Part model, mm, in its own coordinate system. A direction names the side the tool comes from. Give positions to 0.01 mm unless a question says otherwise; leave off trailing zeros. Order: outer loops, then holes, each group sorted by start corner. A loop starts at its lowest first (then second) coordinate and runs counter-clockwise, first axis right, second up. Notation, with made-up numbers: (-17, 54.25) -> (-8, 54.25) arc R15 ccw to (-8, 71.25) -> close; hole circle Ø11 at (-21.75, 80). An arc over 180 degrees is marked (long way). Write item = value, one per line. Start each with the question number.
Item 1: Band-saw the part on C-C on y = 6.25. Write the cut outline in (x, z).
Item 2: Band-saw the part on A-A on y = 3.75. Write the cut outline in (x, z).
Item 3: Pull direction Z, two halves, no side cores. Call faces 1 (the face through (-1, 7, 3)), 2 (the face through (-1, 6, 2)), 3 (the face through (-2, 6.3, 2.4)), 4 (the face through (-15, 6.7, 0.4)): +Z half, -Z half, draft (parallel to the pull), parting line (faces both ways), or undercut.
Item 4: Band-saw the part on B-B on z = 1.7. Write the cut outline in (x, y), plus the area to 3 significant figures.
Item 5: Flat gauge pins, fed straight in: P1, Ø0.9, axis at x = -9, z = 2, coming from the -Y side; P2, Ø1.2, axis at y = 7, z = 2, coming from the -X side. Where does each tip first touch, or does it go through?
Item 6: Band-saw the part on D-D on z = 0.3. Write the cut outline in (x, y), plus the area to 3 significant figures.
Item 7: Tool access for faces 5 (the face through (-9, 4, 0.6)), 6 (the face through (-6, 6, 0)), 7 (the face through (-1, 6, 1)): list every direction of +Z, -Z, +X, -X, +Y, -Y with a clear straight run to the whole face (end or side of a thin tool).
Item 8: Drill centre lines: line 1 along Y through (x, z) = (-8.75, 1.2); line 2 along Z through (x, y) = (-8, 10.5); line 3 along Y through (x, z) = (-9.25, 2.85). Where is each one in solid material? Low to high.
```python
from build123d import *

# Parameters (mm, degrees)
SKETCH1_W           = 15
SKETCH1_H           = 12.5
BOSS_EXTRUDE1_DEPTH = 3
CUT_EXTRUDE1_DEPTH  = 13
SKETCH4_W           = 1
SKETCH4_H           = 9
CUT_EXTRUDE2_DEPTH  = 19.282505299
SKETCH5_R           = 1.9939
CUT_EXTRUDE3_DEPTH  = 1082.289832046


with BuildPart() as part:
    # Sketch1 → Boss-Extrude1 (new body)
    with BuildSketch(Plane.XY):
        with Locations((-7.5, 6.25)):
            Rectangle(SKETCH1_W, SKETCH1_H)
    extrude(amount=BOSS_EXTRUDE1_DEPTH)

    # Sketch3 → Cut-Extrude1 (cut)
    with BuildSketch(Plane.ZY.offset(15)):
        Polygon((0.6, 11.75), (2.4, 11.75), (2.4, 10.75), (3, 10.75), (3, 1.75), (2.4, 1.75), (2.4, 0.75), (0.6, 0.75), align=None)
    extrude(amount=-CUT_EXTRUDE1_DEPTH, mode=Mode.SUBTRACT)

    # Sketch4 → Cut-Extrude2 (cut, through all)
    with BuildSketch(Plane.ZY.offset(2)):
        with Locations((1.5, 6.25)):
            Rectangle(SKETCH4_W, SKETCH4_H)
    extrude(amount=-CUT_EXTRUDE2_DEPTH, mode=Mode.SUBTRACT)

    # Sketch5 → Cut-Extrude3 (cut, through all)
    with BuildSketch(Plane(origin=(-632.3963488, -864.572858382, 0.6), x_dir=(1, 0, 0), z_dir=(0, 0, 1))):
        with Locations((623.8939488, 870.822858382)):
            Circle(SKETCH5_R)
    extrude(amount=-CUT_EXTRUDE3_DEPTH, mode=Mode.SUBTRACT)


solid = part.part
```
Values found:
q1.outline = (-15, 0) -> (-10.5, 0) -> (-10.5, 0.6) -> (-15, 0.6) -> close; (-6.51, 0) -> (0, 0) -> (0, 1) -> (-2, 1) -> (-2, 0.6) -> (-6.51, 0.6) -> close; (-2, 2) -> (0, 2) -> (0, 3) -> (-2, 3) -> close
q2.outline = (-15, 0) -> (0, 0) -> (0, 1) -> (-2, 1) -> (-2, 0.6) -> (-15, 0.6) -> close; (-2, 2) -> (0, 2) -> (0, 3) -> (-2, 3) -> close
q3.face_1 = +Z half
q3.face_2 = undercut
q3.face_3 = undercut
q3.face_4 = draft
q4.outline = (-15, 0) -> (0, 0) -> (0, 1.75) -> (-2, 1.75) -> (-2, 0.75) -> (-15, 0.75) -> close; (-15, 11.75) -> (-2, 11.75) -> (-2, 10.75) -> (0, 10.75) -> (0, 12.5) -> (-15, 12.5) -> close
q4.area = 26.5 mm^2
q5.P1 = 0
q5.P2 = -2
q6.outline = (-15, 0) -> (0, 0) -> (0, 12.5) -> (-15, 12.5) -> close; hole circle Ø3.99 at (-8.5, 6.25)
q6.area = 175 mm^2
q7.face_5 = -X
q7.face_6 = -Z, +X, -X, +Y, -Y
q7.face_7 = +X, -X
q8.line_1 = 0 to 0.75, 11.75 to 12.5
q8.line_2 = 0 to 0.6
q8.line_3 = 0 to 1.75, 10.75 to 12.5
